from build123d import *

# Parameters (mm, degrees)
SKETCH1_W                                  = 600
SKETCH1_H                                  = 500
BOSS_EXTRUDE1_DEPTH                        = 175
SHELL1_T                                   = 10
SKETCH3_W                                  = 620
SKETCH3_H                                  = 360
BOSS_EXTRUDE2_DEPTH                        = 20
SKETCH5_W                                  = 120
SKETCH5_H                                  = 150
CUT_EXTRUDE1_DEPTH                         = 50
BOSS_EXTRUDE3_DEPTH                        = 15
SKETCH9_R                                  = 10
SKETCH9_R_2                                = 8.804977656
SKETCH9_R_3                                = 9.206937975
BOSS_EXTRUDE4_DEPTH                        = 180
BOSS_EXTRUDE8_START                        = -260
BOSS_EXTRUDE8_DEPTH                        = 10
SKETCH147_W                                = 600
SKETCH147_H                                = 15
CUT_EXTRUDE2_DEPTH                         = 10
SKETCH148_R                                = 3.5
BOSS_EXTRUDE10_DEPTH                       = 600
SKETCH149_R                                = 9
CUT_EXTRUDE3_DEPTH                         = 7
MIRROR3_AT_THE_SECOND_PLANE_COPY_1_SKETC_R = 9
MIRROR3_AT_THE_SECOND_PLANE_COPY_1_DEPTH   = 7
SKETCH150_W                                = 60
SKETCH150_H                                = 10
CUT_EXTRUDE4_DEPTH                         = 30
SKETCH155_W                                = 290.489530142
SKETCH155_H                                = 28
CUT_EXTRUDE11_DEPTH                        = 716.53321378
BOSS_EXTRUDE11_DEPTH                       = 488
BOSS_EXTRUDE12_DEPTH                       = 125
BOSS_EXTRUDE12_DEPTH_BACK                  = 445
SKETCH160_W                                = 600
SKETCH160_H                                = 500
CUT_EXTRUDE12_DEPTH                        = 8
SKETCH161_W                                = 618
SKETCH161_H                                = 137.7775458
BOSS_EXTRUDE13_DEPTH                       = 28


with BuildPart() as part:
    # Sketch1 → Boss-Extrude1 (new, symmetric)
    with BuildSketch(Plane.XY):
        Rectangle(SKETCH1_W, SKETCH1_H)
    extrude(amount=BOSS_EXTRUDE1_DEPTH, both=True)

    # Shell1
    shell1_openings = [part.faces().sort_by_distance(p)[0] for p in [
        (0, 0, 175),
    ]]
    offset(amount=SHELL1_T, openings=shell1_openings, kind=Kind.INTERSECTION)

    # Sketch3 → Boss-Extrude2 (add)
    with BuildSketch(Plane.XZ.offset(260)):
        with Locations((0, -5)):
            Rectangle(SKETCH3_W, SKETCH3_H)
    extrude(amount=BOSS_EXTRUDE2_DEPTH)

    # Sketch5 → Cut-Extrude1 (cut)
    with BuildSketch(Plane.XZ.offset(280)):
        with Locations((-170, 100)):
            Rectangle(SKETCH5_W, SKETCH5_H)
        with Locations((170, 100)):
            Rectangle(SKETCH5_W, SKETCH5_H)
        with Locations((-220, -185)):
            Rectangle(SKETCH5_W, SKETCH5_H)
        with Locations((220, -185)):
            Rectangle(SKETCH5_W, SKETCH5_H)
    extrude(amount=-CUT_EXTRUDE1_DEPTH, mode=Mode.SUBTRACT)

    # Sketch8 → Boss-Extrude3 (add, symmetric)
    with BuildSketch(Plane(origin=(0, 0, 0), x_dir=(1, 0, 0), z_dir=(0, 1, 0))):
        Polygon((-310, 10), (-315, 10), (-315, -10), (-310, -10), (-310, -15), (-320, -15), (-320, 15), (-310, 15), align=None)
    boss_extrude3 = extrude(amount=BOSS_EXTRUDE3_DEPTH, both=True)

    # Sketch9 → Boss-Extrude4 (add)
    # profile 1 of 2: a face of its own
    with BuildSketch(Plane.ZY.offset(110)):
        with Locations(Location((155, -265, 0), (0, 0, 180))):
            Circle(SKETCH9_R)
        with Locations((155, -265)):
            Circle(SKETCH9_R_2, mode=Mode.SUBTRACT)
    # profile 2 of 2: a face of its own
    with BuildSketch(Plane.ZY.offset(110)):
        with Locations(Location((-165, -265, 0), (0, 0, 180))):
            Circle(SKETCH9_R)
        with Locations(Location((-165, -265, 0), (0, 0, 180))):
            Circle(SKETCH9_R_3, mode=Mode.SUBTRACT)
    boss_extrude4 = extrude(amount=BOSS_EXTRUDE4_DEPTH)

    # Mirror1: Boss-Extrude3, Boss-Extrude4 across plane
    add(boss_extrude3.mirror(Plane(origin=(0, 0, 0), x_dir=(0, 0, 1), z_dir=(1, 0, 0))))
    add(boss_extrude4.mirror(Plane(origin=(0, 0, 0), x_dir=(0, 0, 1), z_dir=(1, 0, 0))))

    # Sketch17 → Boss-Extrude8 (add, symmetric)
    with BuildSketch(Plane(origin=(0, 260, 0), x_dir=(1, 0, 0), z_dir=(0, 1, 0)).offset(BOSS_EXTRUDE8_START)):
        Polygon((-194.223256177, 185), (-204.223256177, 185), (-204.223256177, 191.540544069), (-159.461030104, 191.540544069), (-159.461030104, 185), (-169.461030104, 185), (-169.461030104, 188.442858537), (-194.223256177, 188.442858537), align=None)
        Polygon((194.223256177, 188.442858537), (194.223256177, 185), (204.223256177, 185), (204.223256177, 191.540544069), (159.461030104, 191.540544069), (159.461030104, 185), (169.461030104, 185), (169.461030104, 188.442858537), align=None)
    extrude(amount=BOSS_EXTRUDE8_DEPTH, both=True)

    # Sketch147 → Cut-Extrude2 (cut)
    with BuildSketch(Plane(origin=(0, 260, 0), x_dir=(1, 0, 0), z_dir=(0, 1, 0))):
        with Locations((0, -167.5)):
            Rectangle(SKETCH147_W, SKETCH147_H)
    extrude(amount=-CUT_EXTRUDE2_DEPTH, mode=Mode.SUBTRACT)

    # Sketch148 → Boss-Extrude10 (add)
    with BuildSketch(Plane(origin=(-300, 0, 0), x_dir=(0, 0, -1), z_dir=(1, 0, 0))):
        with Locations(Location((-168, 255, 0), (0, 0, 180))):
            Circle(SKETCH148_R)
    extrude(amount=BOSS_EXTRUDE10_DEPTH)

    # Sketch149 → Cut-Extrude3 (cut)
    with BuildSketch(Plane(origin=(0, 260, 0), x_dir=(1, 0, 0), z_dir=(0, 1, 0))):
        with Locations(Location((-70, 40, 0), (0, 0, 270))):
            Circle(SKETCH149_R)
    cut_extrude3 = extrude(amount=-CUT_EXTRUDE3_DEPTH, mode=Mode.SUBTRACT)

    # Mirror3: Cut-Extrude3 across plane
    add(cut_extrude3.mirror(Plane.XY), mode=Mode.SUBTRACT)

    # Mirror3 at the second plane: Cut-Extrude3 across plane
    add(cut_extrude3.mirror(Plane(origin=(0, 0, 0), x_dir=(0, 0, 1), z_dir=(1, 0, 0))), mode=Mode.SUBTRACT)

    # Mirror3 at the second plane copy 1 sketc → Mirror3 at the second plane copy 1 (cut)
    with BuildSketch(Plane(origin=(0, 260, 0), x_dir=(-1, 0, 0), z_dir=(0, 1, 0))):
        with Locations(Location((-70, 40, 0), (0, 0, 270))):
            Circle(MIRROR3_AT_THE_SECOND_PLANE_COPY_1_SKETC_R)
    extrude(amount=-MIRROR3_AT_THE_SECOND_PLANE_COPY_1_DEPTH, mode=Mode.SUBTRACT)

    # Sketch150 → Cut-Extrude4 (cut)
    with BuildSketch(Plane.XY.offset(175)):
        with Locations((0, -259)):
            Rectangle(SKETCH150_W, SKETCH150_H)
    extrude(amount=-CUT_EXTRUDE4_DEPTH, mode=Mode.SUBTRACT)

    # Sketch155 → Cut-Extrude11 (cut, through all)
    with BuildSketch(Plane.ZY.offset(310)):
        with Locations((0, -266)):
            Rectangle(SKETCH155_W, SKETCH155_H)
    extrude(amount=-CUT_EXTRUDE11_DEPTH, mode=Mode.SUBTRACT)

    # Sketch157 → Boss-Extrude11 (add)
    with BuildSketch(Plane(origin=(-230, 0, 0), x_dir=(0, 0, -1), z_dir=(1, 0, 0))):
        Polygon((-145.244765071, -252), (-175, -252), (-175, -250), (-25, -250), (-25, -252), align=None)
    extrude(amount=BOSS_EXTRUDE11_DEPTH)

    # Sketch159 → Boss-Extrude12 (add, two sides: drawn at the far end of the back side and taken through both)
    with BuildSketch(Plane(origin=(160, 0, 0), x_dir=(0, 0, -1), z_dir=(1, 0, 0)).offset(-BOSS_EXTRUDE12_DEPTH_BACK)):
        Polygon((145.244765071, -252), (185, -252), (185, -230), (175, -230), (175, -250), (110, -250), (110, -252), align=None)
    extrude(amount=BOSS_EXTRUDE12_DEPTH + BOSS_EXTRUDE12_DEPTH_BACK)

    # Sketch160 → Cut-Extrude12 (cut)
    with BuildSketch(Plane.XY.offset(-175)):
        Rectangle(SKETCH160_W, SKETCH160_H)
    extrude(amount=-CUT_EXTRUDE12_DEPTH, mode=Mode.SUBTRACT)

    # Sketch161 → Boss-Extrude13 (add)
    with BuildSketch(Plane.XZ.offset(252)):
        Rectangle(SKETCH161_W, SKETCH161_H)
    extrude(amount=BOSS_EXTRUDE13_DEPTH)


solid = part.part
For this review, take the finished solid that the model builds, in its own axes (mm). A direction names the side the tool comes from. Give positions to 0.01 mm unless a question says otherwise; leave off trailing zeros. Order: outer loops, then holes, each group sorted by start corner. A loop starts at its lowest first (then second) coordinate and runs counter-clockwise, first axis right, second up. Notation, with made-up numbers: (6.25, -7) - (58.25, -7) arc R7 cw to (58.25, 2) - close; hole circle Ø7 at (89.5, 46). An arc over 180 degrees is marked (long way). Answer as a JSON object with one key per item and string values. Group by question number.
Item 1: Take a section at A-A on x = -254.5. Give the boundary of the cut face in (y, z).
Item 2: Take a section at B-B on z = 92.5. Give the boundary of the cut face in (x, y), and give its area (3 significant figures).
Item 3: Draft analysis for pull direction X (two halves, no side actions). For faces 1 (the flat face through (-70, 253, 40)), 2 (the flat face through (0, -264, 160)), 3 (the flat face through (269, -280, 160)), 4 (the flat face through (-320, 0, 0)), state which applies: pulls with the +X half, pulls with the -X half, needs draft (parallel to the pull), parting line crosses it, or undercut.
Item 4: Wall thickness on line 1 along Y through (x, z) = (-252, -165); line 2 along X through (y, z) = (255, 40); line 3 along X through (y, z) = (146.5, 132): over which ranges is each line inside the solid? List them lowest first.
Item 5: Take a section at C-C on y = 123. Give the boundary of the cut face in (x, z).
Item 6: Machinability: for faces 5 (the flat face through (295, -266, -145.245)), 6 (the cylindrical face through (-219.16, -261.17, -174.237)), 7 (the flat face through (-315, 0, 0)), which of the approach directions +Z, -Z, +X, -X, +Y, -Y give a long, thin tool a straight path to every point of the face, cutting with its end or side? Answer none if there is none.
Item 7: Take a section at D-D on x = -70. Give the boundary of the cut face in (y, z), and give its area (3 significant figures).
Item 8: Clearance check with flat-ended pins moving along their axes: pin 1 Ø2 at (x, y) = (-156.5, -28.5) entering from +Z; pin 2 Ø11 at (x, z) = (-313.5, 3) entering from -Y; pin 3 Ø5.5 at (x, y) = (-311.5, 2) entering from -Z; pin 4 Ø8 at (x, z) = (-87.5, -85.5) entering from -Y. State where each tip first meets the part, or that it passes through.
Reported:
{
 "1": {"outline": "(-280, -68.89) - (-252, -68.89) - (-252, -185) - (260, -185) - (260, 160) - (250, 160) - (250, -183) - (-250, -183) - (-250, 175) - (-280, 175) - (-280, 145.24) - (-252, 145.24) - (-252, 68.89) - (-280, 68.89) - close; circle Ø20 at (-265, -165); circle Ø7 at (255, 168); hole circle Ø18.41 at (-265, -165)"},
 "2": {"outline": "(-310, -252) - (310, -252) - (310, 260) - (-310, 260) - close; hole (-300, -250) - (300, -250) - (300, 250) - (-300, 250) - close", "area": "17,400 mm^2"},
 "3": {"face 1": "undercut", "face 2": "undercut", "face 3": "needs draft", "face 4": "pulls with the -X half"},
 "4": {"line 1": "-275 to -274.21, -255.79 to -255, -252 to -250, 250 to 260", "line 2": "-310 to -79, -61 to 61, 79 to 310", "line 3": "-310 to -300, 300 to 310"},
 "5": {"outline": "(-310, -185) - (310, -185) - (310, 175) - (300, 175) - (300, -183) - (-300, -183) - (-300, 175) - (-310, 175) - close"},
 "6": {"face 5": "+X, -X, -Y", "face 6": "none", "face 7": "+Y, -Y"},
 "7": {"outline": "(-280, -185) - (260, -185) - (260, -49) - (253, -49) - (253, -31) - (260, -31) - (260, 31) - (253, 31) - (253, 49) - (260, 49) - (260, 160) - (250, 160) - (250, -183) - (-250, -183) - (-250, 175) - (-280, 175) - (-280, 145.24) - (-252, 145.24) - (-252, 68.89) - (-280, 68.89) - (-280, -68.89) - (-252, -68.89) - (-252, -145.24) - (-280, -145.24) - close; circle Ø7 at (255, 168)", "area": "10,800 mm^2"},
 "8": {"pin 1": "z = -183", "pin 2": "y = -280", "pin 3": "z = -185", "pin 4": "y = -252"}
}
